Can you work these out from the drawing? Everything is in mm from the part's minimum corner. Coordinates: 2 decimals unless noted, no trailing zeros. Loops run counter-clockwise (first coordinate to the right, second up) from the corner with the lowest first, then second, coordinate; pieces in that order, holes last.
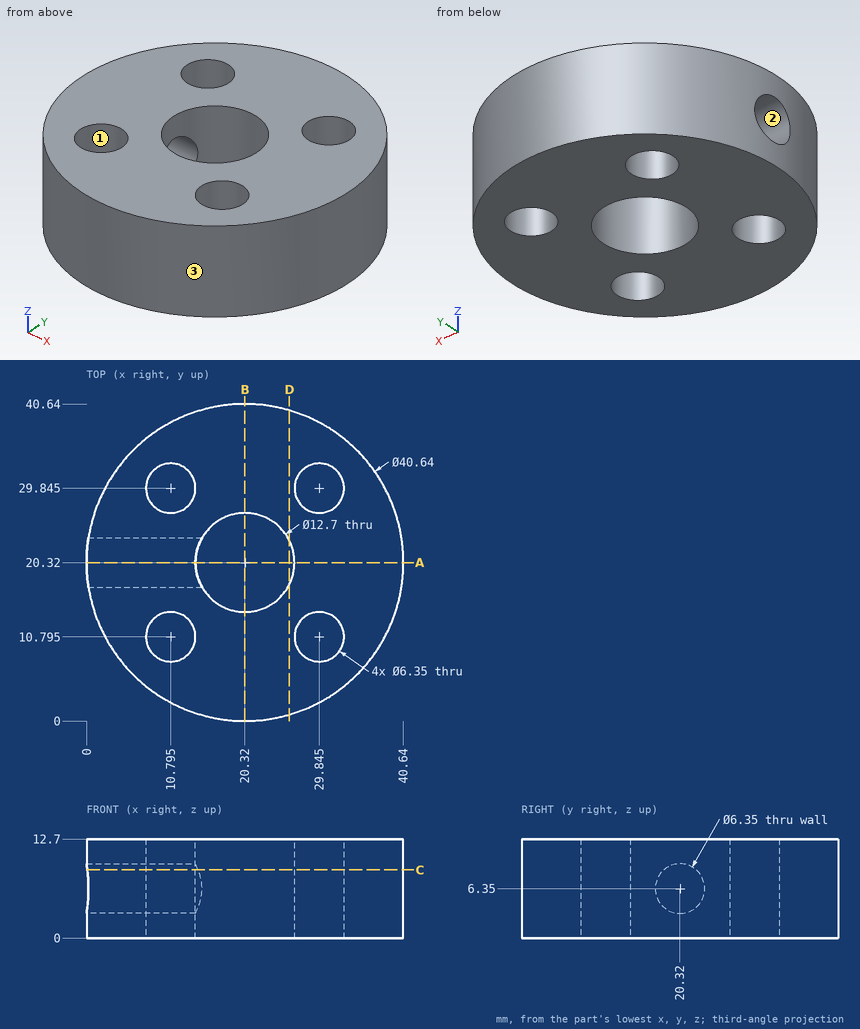
(1) Imagine slicing it at C-C, the plane z = 8.75. Write out the boundary of the cut face in (x, y) (3 decimals), and give its area (3 significant figures).
Answers:
outline: (0.107, 18.241) arc R20.32 ccw (long way) to (0.107, 22.399) - (14.32, 22.399) arc R6.35 cw (long way) to (14.32, 18.241) - close; hole circle Ø6.35 at (10.795, 10.795); hole circle Ø6.35 at (10.795, 29.845); hole circle Ø6.35 at (29.845, 10.795); hole circle Ø6.35 at (29.845, 29.845)
area: 985 mm2
(2) For pin 1 (1 mm diameter, centred on y = 9.5, z = 2.5, fed in from +X); pin 2 (1 mm diameter, centred on y = 7, z = 7.5, fed in from -X); pin 3 (3 mm diameter, centred on y = 36.5, z = 8.5, fed in from -X), each with a flat end and sliding along its axis, tell me the tip position at first contact or that it passes through.
Answers:
pin 1: stops at x = 37.82
pin 2: stops at x = 4.55
pin 3: stops at x = 6.27
(3) We'd pull the mould along X, two halves only. Please class the marked faces 1, 2 and 3: +X half, -X half, draft (parallel to the pull), parting line (faces both ways), or undercut.
Answers:
face 1: undercut
face 2: draft
face 3: parting line
(4) Imagine slicing it at B-B, the plane x = 20.32. Write out the boundary of the cut face in (y, z).
Answers:
outline: (0, 0) - (13.97, 0) - (13.97, 12.7) - (0, 12.7) - close; (26.67, 0) - (40.64, 0) - (40.64, 12.7) - (26.67, 12.7) - close
(5) Imagine slicing it at D-D, the plane x = 26. Write out the boundary of the cut face in (y, z), and give its area (3 significant figures).
Answers:
outline: (0.81, 0) - (17.48, 0) - (17.48, 12.7) - (0.81, 12.7) - close; (23.16, 0) - (39.83, 0) - (39.83, 12.7) - (23.16, 12.7) - close
area: 423 mm2
(6) Imagine slicing it at A-A, the plane y = 20.32. Write out the boundary of the cut face in (x, z) (3 decimals), and give its area (3 significant figures).
Answers:
outline: (0, 0) - (13.97, 0) - (13.97, 3.175) - (0, 3.175) - close; (0, 9.525) - (13.97, 9.525) - (13.97, 12.7) - (0, 12.7) - close; (26.67, 0) - (40.64, 0) - (40.64, 12.7) - (26.67, 12.7) - close
area: 266 mm2
(7) I need wall thicknesses on probe 1 along X at (y, z) = (31, 9.5); probe 2 along X at (y, z) = (10.5, 2.25). Which ranges of each line are inside material? Lowest first, please.
Answers:
probe 1: x = 3.03 to 7.84, 13.75 to 26.89, 32.8 to 37.61
probe 2: x = 2.53 to 7.63, 13.96 to 26.68, 33.01 to 38.11
